from build123d import *

# Parameters (mm, degrees)
CROQUIS1_W            = 50.8
CROQUIS1_H            = 6.31
CROQUIS2_R            = 6.5
CORTAR_EXTRUIR1_DEPTH = 10
CROQUIS5_R            = 6.5
CORTAR_EXTRUIR4_DEPTH = 10
CROQUIS7_W            = 59.2
CROQUIS7_H            = 50.8
CORTAR_EXTRUIR5_DEPTH = 6.31
CROQUIS9_W            = 50.8
CROQUIS9_H            = 66.2
CORTAR_EXTRUIR7_DEPTH = 10
CROQUIS10_R           = 4.7625
CORTAR_EXTRUIR8_DEPTH = 10


with BuildPart() as part:
    # Barrer1: sweep along a curve in space
    with BuildLine() as barrer1_path:
        Line((0, 0, 0), (0, 0, 891.73))
        Line((0, 0, 891.73), (0, -67.38, 891.73))
        Line((0, -67.38, 891.73), (-84.6, -67.38, 891.73))
    # Croquis1 → Barrer1 (sweep)
    with BuildSketch(Plane.XY):
        Rectangle(CROQUIS1_W, CROQUIS1_H)
    sweep(path=barrer1_path.line, transition=Transition.RIGHT)

    # Croquis2 → Cortar-Extruir1 (cut)
    with BuildSketch(Plane(origin=(0, 3.155, 0), x_dir=(1, 0, 0), z_dir=(0, 1, 0))):
        with Locations(Location((0, -16.5, 0), (0, 0, 270))):
            Circle(CROQUIS2_R)
        with Locations(Location((0, -47.5, 0), (0, 0, 270))):
            Circle(CROQUIS2_R)
    extrude(amount=-CORTAR_EXTRUIR1_DEPTH, mode=Mode.SUBTRACT)

    # Croquis5 → Cortar-Extruir4 (cut)
    with BuildSketch(Plane(origin=(0, 0, 888.575), x_dir=(-1, 0, 0), z_dir=(0, 0, -1))):
        with Locations((60, -67.38)):
            Circle(CROQUIS5_R)
    extrude(amount=-CORTAR_EXTRUIR4_DEPTH, mode=Mode.SUBTRACT)

    # Croquis7 → Cortar-Extruir5 (cut)
    with BuildSketch(Plane(origin=(0, 0, 888.575), x_dir=(-1, 0, 0), z_dir=(0, 0, -1))):
        with Locations((55, -67.38)):
            Rectangle(CROQUIS7_W, CROQUIS7_H)
    extrude(amount=-CORTAR_EXTRUIR5_DEPTH, mode=Mode.SUBTRACT)

    # Croquis9 → Cortar-Extruir7 (cut)
    with BuildSketch(Plane(origin=(0, 3.155, 0), x_dir=(1, 0, 0), z_dir=(0, 1, 0))):
        with Locations((0, -33.1)):
            Rectangle(CROQUIS9_W, CROQUIS9_H)
    extrude(amount=-CORTAR_EXTRUIR7_DEPTH, mode=Mode.SUBTRACT)

    # Croquis10 → Cortar-Extruir8 (cut)
    with BuildSketch(Plane(origin=(0, 3.155, 0), x_dir=(1, 0, 0), z_dir=(0, 1, 0))):
        with Locations(Location((0, -91.6, 0), (0, 0, 270))):
            Circle(CROQUIS10_R)
    extrude(amount=-CORTAR_EXTRUIR8_DEPTH, mode=Mode.SUBTRACT)


solid = part.part
Work out the finished part from the listing and answer in its coordinate system (mm). A direction names the side the tool comes from. Round coordinates to 2 decimals unless told otherwise and drop trailing zeros. Order: outer loops, then holes, each group sorted by start corner. A loop starts at its lowest first (then second) coordinate and runs counter-clockwise, first axis right, second up. Notation, with made-up numbers: M 28,-15 L 59,-15 A9 ccw 59,-8 Z; hole C 27,-31 d1. An arc over 180 degrees is marked long. Put each result on its own line as item: value. Start each with the question number.
Q1. Section B-B, the plane y = -58 is taken. Write down the section's boundary in (x, z) (3 decimals), and give its area (3 significant figures).
Q2. Section C-C, the plane z = 340 is taken. Write down the section's boundary in (x, y) (3 decimals), and give its area (3 significant figures).
Q3. Straight lines are drawn through the part: L1, parallel to X at y = 0.5, z = 91.6; L2, parallel to X at y = -1, z = 91; L3, parallel to Z at x = -12, y = -15 (3 decimals). For each, find the intervals that lie inside material, in ascending order. Write a range as [from, to].
Q4. A flat-ended cylindrical pin translates along its axis: pin 1 (1.5 mm diameter, centred on x = -4, y = -48, fed in from -Z) (3 decimals). Find the tip coordinate at first contact, or state that the pin passes through.
Q5. A tool of negligible diameter and unlimited length cuts with its end or side. For faces 1 (the flat face through (0, -3.155, 483)), 2 (the flat face through (25.4, -2, 482)), from which of +Z, -Z, +X, -X, +Y, -Y can it reach the whole face along a straight path? Write none if from no direction.
Q6. Section A-A, the plane x = -14 is taken. Write down the section's boundary in (y, z) (3 decimals).
Findings below:
1. outline: M -25.4,888.575 L 25.4,888.575 L 25.4,894.885 L -25.4,894.885 Z
1. area: 321 mm^2
2. outline: M -25.4,-3.155 L 25.4,-3.155 L 25.4,3.155 L -25.4,3.155 Z
2. area: 321 mm^2
3. L1: x = [-25.4, -4.76], [4.76, 25.4]
3. L2: x = [-25.4, -4.72], [4.72, 25.4]
3. L3: z = [888.575, 894.885]
4. pin 1: stops at z = 888.575
5. face 1: -Z, +X, -X, -Y
5. face 2: +Z, -Z, +X, +Y, -Y
6. outline: M -92.78,888.575 L -3.155,888.575 L -3.155,66.2 L 3.155,66.2 L 3.155,894.885 L -92.78,894.885 Z
